Geometry check sheet. Reference: the model listing, model coordinates, mm. Round coordinates to 2 decimals unless told otherwise and drop trailing zeros. Loops run counter-clockwise (first coordinate to the right, second up) from the corner with the lowest first, then second, coordinate; pieces in that order, holes last. Notation, with made-up numbers: (46, -15) -> (104, -15) arc R25 cw to (104, -2) -> close; hole circle Ø2 at (59.25, 68.25). An arc over 180 degrees is marked (long way). Use one line per item in the form item = value.
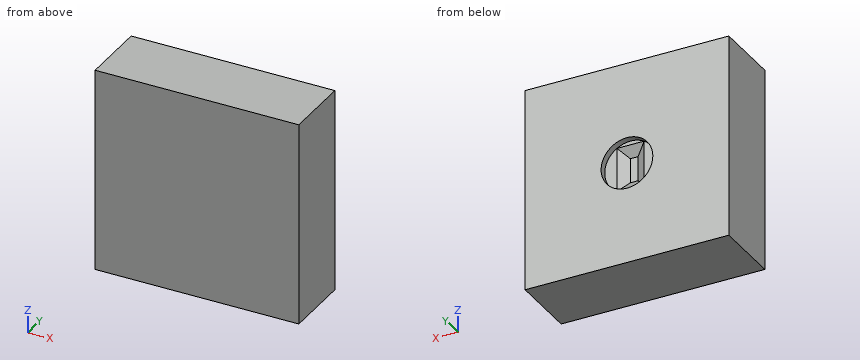
from build123d import *

# Parameters (mm, degrees)
SKETCH1_W           = 30
SKETCH1_H           = 30
BOSS_EXTRUDE1_DEPTH = 10
SKETCH2_R           = 3.81
BORE_DEPTH          = 1
SKETCH3_W           = 4
SKETCH3_H           = 6.485707364
GROOVE_DEPTH        = 1
GROOVE_DRAFT        = -55


with BuildPart() as part:
    # Sketch1 → Boss-Extrude1 (new body)
    with BuildSketch(Plane(origin=(0, 0, 0), x_dir=(1, 0, 0), z_dir=(0, 1, 0))):
        Rectangle(SKETCH1_W, SKETCH1_H)
    extrude(amount=BOSS_EXTRUDE1_DEPTH)

    # Sketch2 → bore (cut)
    with BuildSketch(Plane(origin=(0, 10, 0), x_dir=(1, 0, 0), z_dir=(0, 1, 0))):
        with Locations(Location((0, 0, 0), (0, 0, 270))):
            Circle(SKETCH2_R)
    extrude(amount=-BORE_DEPTH, mode=Mode.SUBTRACT)


with BuildPart() as groove_tool:
    # Sketch3 → groove (with draft: the straight prism first)
    with BuildSketch(Plane(origin=(0, 9, 0), x_dir=(1, 0, 0), z_dir=(0, 1, 0))):
        Rectangle(SKETCH3_W, SKETCH3_H)
    extrude(amount=-GROOVE_DEPTH)
    # groove: the draft: its side faces are tilted about the plane it starts from
    groove_sides = [groove_tool.faces().sort_by_distance(p)[0] for p in [
        (-2, 8.5, 0),
        (0, 8.5, 3.242853682),
        (2, 8.5, 0),
        (0, 8.5, -3.242853682),
    ]]
    draft(groove_sides, Plane(origin=(0, 9, 0), x_dir=(1, 0, 0), z_dir=(0, 1, 0)), GROOVE_DRAFT)


with BuildPart() as part_1:
    add(part.part)

    # groove: cut by groove_tool
    add(groove_tool.part, mode=Mode.SUBTRACT)


solid = part_1.part
1. Gauge pin test, flat ends, axial feed: pin 1 (4.5 mm diameter, centred on x = 0, z = 0, fed in from +Y); pin 2 (0.9 mm diameter, centred on x = 0, z = -0.5, fed in from +Y). Record the tip position at first contact, or that the pin passes through.
Return value:
pin_1 = 9
pin_2 = 8
2. Section check A-A (x = 0). Record the boundary of the cut face in (y, z), then the cut area to 3 significant figures.
Return value:
outline = (0, -15) -> (10, -15) -> (10, -3.81) -> (9, -3.81) -> (9, -3.24) -> (8, -1.81) -> (8, 1.81) -> (9, 3.24) -> (9, 3.81) -> (10, 3.81) -> (10, 15) -> (0, 15) -> close
area = 287 mm2
3. Material ranges on line 1 along X through (y, z) = (9.2, 0), recorded low to high.
Return value:
line_1 = -15 to -3.81, 3.81 to 15
4. Section check B-B (z = 0). Record the boundary of the cut face in (x, y).
Return value:
outline = (-15, 0) -> (15, 0) -> (15, 10) -> (3.81, 10) -> (3.81, 9) -> (2, 9) -> (0.57, 8) -> (-0.57, 8) -> (-2, 9) -> (-3.81, 9) -> (-3.81, 10) -> (-15, 10) -> close
